```python
from build123d import *

# Parameters (mm, degrees)
CUT_EXTRUDE1_DEPTH = 45.362146026


with BuildPart() as part:
    # Sketch1 → Revolve1 (revolve)
    with BuildSketch(Plane.XY, mode=Mode.PRIVATE) as revolve1_sk:
        Polygon((0, 0), (-4, 0), (-4, -0.6), (-3.8, -0.6), (-3.8, -1.5), (-4, -1.5), (-4, -42.5), (-3.8, -42.5), (-3.8, -43.4), (-4, -43.4), (-4, -44), (0, -44), align=None)
    revolve(revolve1_sk.sketch.rotate(Axis((0, -44, 0), (0, 1, 0)), 270), axis=Axis((0, -44, 0), (0, 1, 0)))

    # Sketch2 → Cut-Extrude1 (cut, through all)
    with BuildSketch(Plane(origin=(0, 0, 0), x_dir=(1, 0, 0), z_dir=(0, 1, 0))):
        with BuildLine():
            Line((2.8, -2.856571371), (2.8, 2.856571371))
            ThreePointArc((2.8, 2.856571371), (4, 0), (2.8, -2.856571371))
        make_face()
    extrude(amount=-CUT_EXTRUDE1_DEPTH, mode=Mode.SUBTRACT)


solid = part.part
```
Geometry: final body of the model. Coordinates: model frame, mm. A direction names the side the tool comes from. Round coordinates to 2 decimals unless told otherwise and drop trailing zeros. Order: outer loops, then holes, each group sorted by start corner. A loop starts at its lowest first (then second) coordinate and runs counter-clockwise, first axis right, second up. Notation, with made-up numbers: (70.25, -10.75) - (123.25, -10.75) arc R20 ccw to (123.25, 20.25) - close; hole circle Ø4 at (-1, -11.5). An arc over 180 degrees is marked (long way). Use CSV: the item, a comma, the result in double quotes. Start each with the question number.
Q1. Section query B-B (y = -27.5). Return loops of the section in (x, z).
Q2. Material intervals for line 1 along X through (y, z) = (-30, 0.25); line 2 along Z through (x, y) = (2.25, -27); line 3 along Z through (x, y) = (-1, -12), sorted ascending. Write a range as from..to.
Q3. Mould query, pull axis Y, two halves, no side actions, for faces 3 (the face through (-3.8, -1.1, -0.1)), 4 (the face through (-1, 0, 0)), 5 (the face through (2.8, -22, 0)). Classes: +Y half, -Y half, draft (parallel to the pull), parting line (faces both ways), or undercut.
Q4. Access query for faces 1 (the face through (-3.8, -43, -0.1)), 2 (the face through (-4, -22, 0)). Directions: +Z, -Z, +X, -X, +Y, -Y. A direction counts if a zero-diameter tool reaches every point of the face in a straight line with its end or side. Return the directions, or none.
Q5. Section query A-A (z = 1.75). Return loops of the section in (x, y).
Q6. First-contact query: pin 1 (2 mm diameter, centred on x = -0.5, z = 1.5, fed in from +Y). Flat tip, straight axial feed; report the tip coordinate or a pass-through.
Result set:
1,outline,"(2.8, -2.86) - (2.8, 2.86) arc R4 ccw (long way) to start"
2,line 1,"x = -3.99..2.8"
2,line 2,"z = -3.31..3.31"
2,line 3,"z = -3.87..3.87"
3,face 3,"undercut"
3,face 4,"+Y half"
3,face 5,"draft"
4,face 1,"none"
4,face 2,"+Y, -Y"
5,outline,"(-3.6, -44) - (2.8, -44) - (2.8, 0) - (-3.6, 0) - (-3.6, -0.6) - (-3.37, -0.6) - (-3.37, -1.5) - (-3.6, -1.5) - (-3.6, -42.5) - (-3.37, -42.5) - (-3.37, -43.4) - (-3.6, -43.4) - close"
6,pin 1,"stops at y = 0"
